Can you work these out from the drawing? Everything is in mm from the part's minimum corner. Coordinates: 2 decimals unless noted, no trailing zeros. Loops run counter-clockwise (first coordinate to the right, second up) from the corner with the lowest first, then second, coordinate; pieces in that order, holes last. Notation, with made-up numbers: (69.5, 51.5) - (116.5, 51.5) arc R19 cw to (116.5, 65.5) - close; hole circle Ø5 at (-9.75, 8). An arc over 180 degrees is marked (long way). Put each result on its own line as item: value. Start each with the question number.
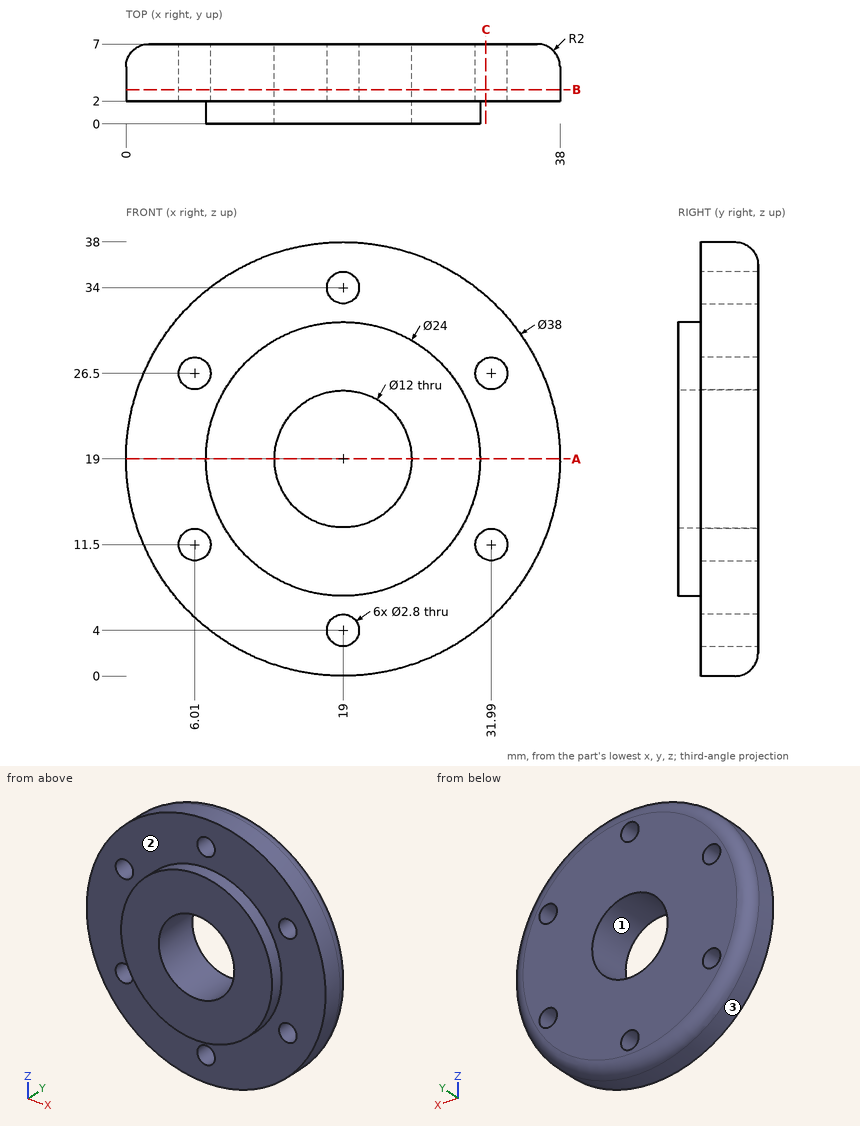
(1) I want a section at C-C on x = 31.5. Count the separate pieces of the cut face and the enclosed holes in it.
(2) I want a section at B-B on y = 3. List the corners of the cut face in (x, z) for me.
(3) For pin 1 Ø3.5 at (x, z) = (31.99, 26.5) entering from -Y; pin 2 Ø1.5 at (y, z) = (2.5, 33.5) entering from -X; pin 3 Ø1 at (y, z) = (5.5, 28) entering from -X, each with a flat end and sliding along its axis, tell me the tip position at first contact or that it passes through.
(4) If we mould it in two halves opening along X, with no side actions, what happens to the marked faces 1, 2 and 3? For each: pulls with the +X half, pulls with the -X half, needs draft (parallel to the pull), parting line crosses it, or undercut.
(5) I want a section at A-A on z = 19. List the corners of the cut face in (x, y) for me.
(6) I need wall thicknesses on L1, parallel to X at y = 4.35, z = 11.5; L2, parallel to X at y = 5.3, z = 26.5; L3, parallel to X at y = 2.75, z = 19. Which ranges of each line are inside material? Lowest first, please. Write a range as [from, to].
Answer sheet:
1. separate pieces: 3
1. enclosed holes: 0
2. outline: circle Ø38 at (19, 19); hole circle Ø2.8 at (6.01, 11.5); hole circle Ø2.8 at (6.01, 26.5); hole circle Ø12 at (19, 19); hole circle Ø2.8 at (19, 4); hole circle Ø2.8 at (19, 34); hole circle Ø2.8 at (31.99, 11.5); hole circle Ø2.8 at (31.99, 26.5)
3. pin 1: stops at y = 2
3. pin 2: stops at x = 5.89
3. pin 3: stops at x = 2.05
4. face 1: undercut
4. face 2: needs draft
4. face 3: parting line crosses it
5. outline: (0, 2) - (7, 2) - (7, 0) - (13, 0) - (13, 7) - (2, 7) arc R2 ccw to (0, 5) - close; (25, 0) - (31, 0) - (31, 2) - (38, 2) - (38, 5) arc R2 ccw to (36, 7) - (25, 7) - close
6. L1: x = [1.54, 4.61], [7.41, 30.59], [33.39, 36.46]
6. L2: x = [1.57, 4.61], [7.41, 30.59], [33.39, 36.43]
6. L3: x = [0, 13], [25, 38]
